Design review of the part built by this model. Coordinates are the model's own, in mm. A direction names the side the tool comes from. Coordinates: 2 decimals unless noted, no trailing zeros. Order: outer loops, then holes, each group sorted by start corner. A loop starts at its lowest first (then second) coordinate and runs counter-clockwise, first axis right, second up. Notation, with made-up numbers: M 37.25,3.5 L 44.25,3.5 A27 ccw 44.25,25.5 Z; hole C -27,36 d3. An arc over 180 degrees is marked long. Use CSV: the item, a comma, the result in double quotes.
```python
from build123d import *

# Parameters (mm, degrees)
SKETCH1_R           = 5
BOSS_EXTRUDE1_DEPTH = 30
SKETCH2_W           = 20
SKETCH2_H           = 44
BOSS_EXTRUDE2_DEPTH = 10
CUT_EXTRUDE2_START  = -5
SKETCH4_W           = 20
SKETCH4_H           = 44
SKETCH4_R           = 5
CUT_EXTRUDE2_DEPTH  = 5


with BuildPart() as part:
    # Sketch1 → Boss-Extrude1 (new body)
    with BuildSketch(Plane(origin=(0, 0, 0), x_dir=(1, 0, 0), z_dir=(0, 1, 0))):
        with Locations(Location((0, 0, 0), (0, 0, 270))):
            Circle(SKETCH1_R)
    extrude(amount=BOSS_EXTRUDE1_DEPTH)

    # Sketch2 → Boss-Extrude2 (add)
    with BuildSketch(Plane(origin=(0, 30, 0), x_dir=(1, 0, 0), z_dir=(0, 1, 0))):
        Rectangle(SKETCH2_W, SKETCH2_H)
    boss_extrude2 = extrude(amount=-BOSS_EXTRUDE2_DEPTH)

    # Sketch4 → Cut-Extrude2 (cut)
    with BuildSketch(Plane(origin=(0, 30, 0), x_dir=(1, 0, 0), z_dir=(0, 1, 0)).offset(CUT_EXTRUDE2_START)):
        Rectangle(SKETCH4_W, SKETCH4_H)
        with Locations(Location((0, 0, 0), (0, 0, 270))):
            Circle(SKETCH4_R, mode=Mode.SUBTRACT)
    cut_extrude2 = extrude(amount=CUT_EXTRUDE2_DEPTH, mode=Mode.SUBTRACT)

    # Mirror2: Boss-Extrude2, Cut-Extrude2 across plane
    add(boss_extrude2.mirror(Plane(origin=(0, 15, 0), x_dir=(0, 0, 1), z_dir=(0, -1, 0))))
    add(cut_extrude2.mirror(Plane(origin=(0, 15, 0), x_dir=(0, 0, 1), z_dir=(0, -1, 0))), mode=Mode.SUBTRACT)


solid = part.part
```
(1) Add section B-B on z = -6. State the section outline as (x, y) points.
The answers:
outline,"M -10,5 L 10,5 L 10,10 L -10,10 Z; M -10,20 L 10,20 L 10,25 L -10,25 Z"
(2) The part is to be moulded in two halves that separate along Y. For faces 3 (the face through (-4.88, 14.93, -1.08)), 4 (the face through (-4.88, 27.46, -1.08)), 5 (the face through (0, 30, 0)), say which applies: pulls with the +Y half, pulls with the -Y half, needs draft (parallel to the pull), parting line crosses it, or undercut.
The answers:
face 3,"undercut"
face 4,"needs draft"
face 5,"pulls with the +Y half"
(3) Wall thickness on probe 1 along Y at (x, z) = (-3, -8); probe 2 along X at (y, z) = (13.25, -2); probe 3 along Z at (x, y) = (-0.5, 13): over which ranges is each line inside the solid? List them lowest first.
The answers:
probe 1,"y = 5 to 10, 20 to 25"
probe 2,"x = -4.58 to 4.58"
probe 3,"z = -4.97 to 4.97"
(4) Clearance check with a flat-ended pin moving along its axis: P1, Ø3, axis at y = 18, z = -12.5, coming from the +X side. State where the tip first meets the part, or that it passes through.
The answers:
P1,"passes through"
(5) For faces 1 (the face through (10, 7, 0)), 2 (the face through (-4.88, 2.54, -1.08)), list the 3-axis set-ups (+Z, -Z, +X, -X, +Y, -Y) from which the entire face can be reached by the end or side of a thin tool; tool diameter is ignored.
The answers:
face 1,"+Z, -Z, +X, +Y, -Y"
face 2,"-Y"
(6) Add section D-D on z = 0. State the section outline as (x, y) points.
The answers:
outline,"M -10,5 L -5,5 L -5,0 L 5,0 L 5,5 L 10,5 L 10,10 L 5,10 L 5,20 L 10,20 L 10,25 L 5,25 L 5,30 L -5,30 L -5,25 L -10,25 L -10,20 L -5,20 L -5,10 L -10,10 Z"
(7) Add section A-A on x = 6.5. State the section outline as (y, z) points, and give its area (3 significant figures).
The answers:
outline,"M 5,-22 L 10,-22 L 10,22 L 5,22 Z; M 20,-22 L 25,-22 L 25,22 L 20,22 Z"
area,"440 mm2"
(8) Add section C-C on x = 0. State the section outline as (y, z) points.
The answers:
outline,"M 0,-5 L 5,-5 L 5,-22 L 10,-22 L 10,-5 L 20,-5 L 20,-22 L 25,-22 L 25,-5 L 30,-5 L 30,5 L 25,5 L 25,22 L 20,22 L 20,5 L 10,5 L 10,22 L 5,22 L 5,5 L 0,5 Z"
